Geometry: final body of the model. Coordinates: model frame, mm. A direction names the side the tool comes from. Coordinates: 2 decimals unless noted, no trailing zeros. Loops run counter-clockwise (first coordinate to the right, second up) from the corner with the lowest first, then second, coordinate; pieces in that order, holes last. Notation, with made-up numbers: (-38, 8) - (-17, 8) arc R26 ccw to (-17, 46) - close; hole circle Ø3 at (38.25, 30). An arc over 180 degrees is marked (long way). Answer in a Markdown table with one row per item.
from build123d import *

# Parameters (mm, degrees)
F0_W          = 78.9395868778
F0_H          = 47.8476444364
F1_DEPTH      = 12.7
F2_R          = 6.35
F3_DEPTH      = 12.7
F5_DEPTH      = 33.02
F6_SIZE       = 25.4
F8_DEPTH      = 5.08
F9_T4_ANGLE   = 53.6437900891
F9_T7_DEPTH   = 53.5623511666
F9_T9_DEPTH   = 53.5623511666
F10_T1_DEPTH  = 85.7200228127
F10_T3_DEPTH  = 177.8
F10_T5_DEPTH  = 85.7200228127
F10_T7_DEPTH  = 177.8
F10_T12_DEPTH = 52.1697934389
F10_T17_DEPTH = 52.1697934389


# Not quite as in the source:
# - a fillet or chamfer that OpenCascade refuses, or shapes differently, is made with other operations: its cross-section is extruded or revolved along the edge and cut away or added


with BuildPart() as f1:
    # F0 (on Front) → F1 (new body)
    with BuildSketch(Plane.XZ):
        Polygon((-39.4697934389, 124.0476444364), (-76.2, 76.2), (-39.4697934389, 76.2), align=None)
        Polygon((-39.4697934389, 76.2), (-76.2, 76.2), (-76.2, -76.2), (76.2, -76.2), (76.2, 76.2), (39.4697934389, 76.2), (39.4697934389, 28.3523555636), (-39.4697934389, 28.3523555636), align=None)
        with Locations((0, 100.1238222182)):
            Rectangle(F0_W, F0_H)
        Polygon((39.4697934389, 124.0476444364), (39.4697934389, 76.2), (76.2, 76.2), align=None)
        with Locations((0, 52.2761777818)):
            Rectangle(F0_W, F0_H)
    extrude(amount=F1_DEPTH)

    # F2 (on face) → F3 (join)
    with BuildSketch(Plane.XZ.offset(12.7)):
        Circle(F2_R)
    extrude(amount=F3_DEPTH)

    # F4 (on face) → F5 (join)
    with BuildSketch(Plane.XZ.offset(12.7)):
        Polygon((0, 124.0476444364), (-19.05, 101.6), (19.05, 101.6), align=None)
        with BuildLine():
            Line((19.05, 101.6), (-19.05, 101.6))
            Line((-19.05, 101.6), (-19.05, 63.5))
            ThreePointArc((-19.05, 63.5), (0, 66.2959463316), (19.05, 63.5))
            Line((19.05, 63.5), (19.05, 101.6))
        make_face()
    extrude(amount=F5_DEPTH)

    # F6
    f6_edges = [f1.edges().sort_by_distance(p)[0] for p in [
        (9.525, -45.72, 112.823822),
        (-9.525, -45.72, 112.823822),
    ]]
    chamfer(f6_edges, length=F6_SIZE)

    # F7 (on face) → F8 (join)
    with BuildSketch(Plane.XZ.offset(45.72)):
        with BuildLine():
            ThreePointArc((7.9480178428, 20.4315265516), (8.0977413026, 21.3227137731), (8.1478546035, 22.225))
            ThreePointArc((8.1478546035, 22.225), (-0.9022862269, 30.3227413026), (-7.9480178428, 20.4315265516))
            ThreePointArc((-7.9480178428, 20.4315265516), (0, 14.0771453965), (7.9480178428, 20.4315265516))
        make_face()
        with BuildLine():
            ThreePointArc((-7.9480178428, 20.4315265516), (-0.9022862269, 30.3227413026), (8.1478546035, 22.225))
            ThreePointArc((8.1478546035, 22.225), (8.0977413026, 21.3227137731), (7.9480178428, 20.4315265516))
            Line((7.9480178428, 20.4315265516), (17.7511165922, 63.8752718956))
            ThreePointArc((17.7511165922, 63.8752718956), (0, 66.2959463316), (-17.7511165922, 63.8752718956))
            Line((-17.7511165922, 63.8752718956), (-7.9480178428, 20.4315265516))
        make_face()
        with BuildLine():
            Line((0, 84.7923718226), (-17.7511165922, 63.8752718956))
            ThreePointArc((-17.7511165922, 63.8752718956), (0, 66.2959463316), (17.7511165922, 63.8752718956))
            Line((17.7511165922, 63.8752718956), (0, 84.7923718226))
        make_face()
    extrude(amount=F8_DEPTH)

    # F9: chamfer of 5.08 on 3 edges, made by hand


with BuildPart() as f9_tool2:
    # F9_s3 → F9_t4 (revolve)
    with BuildSketch(Plane(origin=(0, 0, 0), x_dir=(0, 1, 0), z_dir=(-0.8924134547, 0, -0.4512186011))):
        Polygon((-40.64, -66.2959463316), (-45.72, -61.2159463316), (-45.72, -66.2959463316), align=None)
    revolve(axis=Axis((0, -45.72, 0), (0, 1, 0)), revolution_arc=F9_T4_ANGLE)

    split(bisect_by=Plane(origin=(-3.1759235814, 0, -0.7166484437), x_dir=(0, 1, 0), z_dir=(0.9754736958, 0, 0.2201160349)), keep=Keep.TOP)

    split(bisect_by=Plane(origin=(3.1759235814, 0, -0.7166484437), x_dir=(0, 1, 0), z_dir=(-0.9754736958, 0, 0.2201160349)), keep=Keep.TOP)


with BuildPart() as f1_1:
    add(f1.part)

    # F9_t1: union F9_tool2
    add(f9_tool2.part)

    # F9_s8 → F9_t7 (cut)
    with BuildSketch(Plane(origin=(50.284672357, 0, 59.2531467543), x_dir=(0, 1, 0), z_dir=(-0.6470468375, 0, -0.7624502542))):
        Polygon((-45.72, -54.864636032), (-50.8, -49.784636032), (-50.8, -54.864636032), align=None)
    extrude(amount=F9_T7_DEPTH, mode=Mode.SUBTRACT)

    # F9_s10 → F9_t9 (cut)
    with BuildSketch(Plane(origin=(-15.6273224256, 0, 18.4145184935), x_dir=(0, 1, 0), z_dir=(-0.6470468375, 0, 0.7624502542))):
        Polygon((-45.72, -54.864636032), (-50.8, -49.784636032), (-50.8, -54.864636032), align=None)
    extrude(amount=F9_T9_DEPTH, mode=Mode.SUBTRACT)

    # F10: fillet of radius 5.08 on 7 edges, made by hand

    # F10_s2 → F10_t1 (cut)
    with BuildSketch(Plane(origin=(-0.8185365807, 0, 1.0662898725), x_dir=(0, 1, 0), z_dir=(-0.6089222923, 0, 0.7932298797))):
        with BuildLine():
            ThreePointArc((-12.7, -101.7639955007), (-11.2121024484, -105.3560979491), (-7.62, -106.8439955007))
            Line((-7.62, -106.8439955007), (-12.7, -106.8439955007))
            Line((-12.7, -106.8439955007), (-12.7, -101.7639955007))
        make_face()
    extrude(amount=F10_T1_DEPTH, mode=Mode.SUBTRACT)

    # F10_s4 → F10_t3 (cut)
    with BuildSketch(Plane.XY.offset(-88.9)):
        with BuildLine():
            ThreePointArc((71.12, -12.7), (74.7121024484, -11.2121024484), (76.2, -7.62))
            Line((76.2, -7.62), (76.2, -12.7))
            Line((76.2, -12.7), (71.12, -12.7))
        make_face()
        with BuildLine():
            ThreePointArc((-71.12, -12.7), (-74.7121024484, -11.2121024484), (-76.2, -7.62))
            Line((-76.2, -7.62), (-76.2, -12.7))
            Line((-76.2, -12.7), (-71.12, -12.7))
        make_face()
    extrude(amount=F10_T3_DEPTH, mode=Mode.SUBTRACT)

    # F10_s6 → F10_t5 (cut)
    with BuildSketch(Plane(origin=(53.0153693655, 0, 69.0619732521), x_dir=(0, 1, 0), z_dir=(-0.6089222923, 0, -0.7932298797))):
        with BuildLine():
            ThreePointArc((-12.7, -101.7639955007), (-11.2121024484, -105.3560979491), (-7.62, -106.8439955007))
            Line((-7.62, -106.8439955007), (-12.7, -106.8439955007))
            Line((-12.7, -106.8439955007), (-12.7, -101.7639955007))
        make_face()
    extrude(amount=F10_T5_DEPTH, mode=Mode.SUBTRACT)

    # F10_s8 → F10_t7 (cut)
    with BuildSketch(Plane.YZ.offset(-88.9)):
        with BuildLine():
            ThreePointArc((-12.7, -71.12), (-11.2121024484, -74.7121024484), (-7.62, -76.2))
            Line((-7.62, -76.2), (-12.7, -76.2))
            Line((-12.7, -76.2), (-12.7, -71.12))
        make_face()
    extrude(amount=F10_T7_DEPTH, mode=Mode.SUBTRACT)


with BuildPart() as f10_tool10:
    # F10_s11 → F10_t12 (new body)
    with BuildSketch(Plane.YZ.offset(52.1697934389)):
        with BuildLine():
            ThreePointArc((-12.7, 118.9676444364), (-11.2121024484, 122.5597468848), (-7.62, 124.0476444364))
            Line((-7.62, 124.0476444364), (-12.7, 124.0476444364))
            Line((-12.7, 124.0476444364), (-12.7, 118.9676444364))
        make_face()
    extrude(amount=-F10_T12_DEPTH)

    split(bisect_by=Plane(origin=(61.1977921432, 0, 51.9349789077), x_dir=(0, 1, 0), z_dir=(0.7624502542, 0, 0.6470468375)), keep=Keep.TOP)


with BuildPart() as f1_2:
    add(f1_1.part)

    # F10_t9: cut F10_tool10
    add(f10_tool10.part, mode=Mode.SUBTRACT)


with BuildPart() as f10_tool15:
    # F10_s16 → F10_t17 (new body)
    with BuildSketch(Plane.YZ):
        with BuildLine():
            ThreePointArc((-12.7, 118.9676444364), (-11.2121024484, 122.5597468848), (-7.62, 124.0476444364))
            Line((-7.62, 124.0476444364), (-12.7, 124.0476444364))
            Line((-12.7, 124.0476444364), (-12.7, 118.9676444364))
        make_face()
    extrude(amount=-F10_T17_DEPTH)

    split(bisect_by=Plane(origin=(-61.1977921432, 0, 51.9349789077), x_dir=(0, 1, 0), z_dir=(-0.7624502542, 0, 0.6470468375)), keep=Keep.TOP)


with BuildPart() as f1_3:
    add(f1_2.part)

    # F10_t14: cut F10_tool15
    add(f10_tool15.part, mode=Mode.SUBTRACT)


solid = f1_3.part
(1) Cut plane D-D on y = -32.5. Output: boundary loops of the cut face in (x, z).
Verdict:
| item | result |
|---|---|
| outline | (-19.05, 63.5) arc R66.3 cw to (19.05, 63.5) - (19.05, 82.78) - (0, 105.22) - (-19.05, 82.78) - close |
(2) Cut plane C-C on z = 70.5. Output: boundary loops of the cut face in (x, y).
Verdict:
| item | result |
|---|---|
| outline | (-76.2, -7.62) arc R5.08 ccw to (-71.12, -12.7) - (-19.05, -12.7) - (-19.05, -40.44) - (-5.47, -50.8) - (5.47, -50.8) - (19.05, -40.44) - (19.05, -12.7) - (71.12, -12.7) arc R5.08 ccw to (76.2, -7.62) - (76.2, 0) - (-76.2, 0) - close |
(3) Access query for faces 5 (the face through (0, -25.4, 0)), 6 (the face through (19.05, -25, 78)), 7 (the face through (-0.15, -48.22, 14.08)). Directions: +Z, -Z, +X, -X, +Y, -Y. A direction counts if a zero-diameter tool reaches every point of the face in a straight line with its end or side. Return the directions, or none.
Verdict:
| item | result |
|---|---|
| face 5 | -Z, +X, -X, -Y |
| face 6 | +Z, -Z, +X, -Y |
| face 7 | -Z, -Y |
(4) First-contact query: pin 1 Ø3 at (x, z) = (39, 74.5) entering from -Y; pin 2 Ø4 at (y, z) = (-22.5, 90) entering from +X; pin 3 Ø10 at (x, z) = (-0.5, 2.5) entering from -Y; pin 4 Ø16.5 at (x, z) = (-5, 29.5) entering from +Y. Flat tips, straight axial feed; report the tip coordinate or a pass-through.
Verdict:
| item | result |
|---|---|
| pin 1 | stops at y = -12.7 |
| pin 2 | stops at x = 19.05 |
| pin 3 | stops at y = -25.4 |
| pin 4 | stops at y = 0 |
(5) Pull-direction query (Z, two-part tool) for faces 1 (the face through (-19.46, -11.25, 122.52)), 2 (the face through (-0.271, -25.31, 66.295)), 3 (the face through (0, -50.8, 46)), 4 (the face through (-0.243, -43.78, 63.155)); classes: pulls with the +Z half, pulls with the -Z half, needs draft (parallel to the pull), parting line crosses it, or undercut.
Verdict:
| item | result |
|---|---|
| face 1 | pulls with the +Z half |
| face 2 | undercut |
| face 3 | needs draft |
| face 4 | pulls with the -Z half |
(6) Ray query, probe 1 along Y at (x, z) = (-22, -44); probe 2 along Z at (x, y) = (1, -23); probe 3 along Y at (x, z) = (14.5, 53). Return the intervals inside material, ascending.
Verdict:
| item | result |
|---|---|
| probe 1 | y = -12.7 to 0 |
| probe 2 | z = -6.27 to 6.27, 66.29 to 118.73 |
| probe 3 | y = -50.8 to -45.72, -12.7 to 0 |
(7) Cut plane A-A on z = -17. Output: boundary loops of the cut face in (x, y).
Verdict:
| item | result |
|---|---|
| outline | (-76.2, -7.62) arc R5.08 ccw to (-71.12, -12.7) - (71.12, -12.7) arc R5.08 ccw to (76.2, -7.62) - (76.2, 0) - (-76.2, 0) - close |
(8) Cut plane B-B on y = -5. Output: boundary loops of the cut face in (x, z).
Verdict:
| item | result |
|---|---|
| outline | (-76.2, -76.2) - (76.2, -76.2) - (76.2, 76.2) - (39.47, 124.05) - (-39.47, 124.05) - (-76.2, 76.2) - close |
